```python
from build123d import *

# Parameters (mm, degrees)
SKETCH_1_R           = 30
SKETCH_1_R_2         = 20
EXTRUDE_1_DEPTH      = 30
SKETCH_2_W           = 140
SKETCH_2_H           = 60
EXTRUDE_2_DEPTH      = 10
SKETCH_3_R           = 10
CUT_EXTRUDE_1_DEPTH  = 178.200451467
FILLET_1_RADIUS      = 30
FILLET_1_LENGTH      = 20
EXTRUDE_3_REACH      = 148.287
EXTRUDE_3_END_RADIUS = 30
SKETCH_4_W           = 20
SKETCH_4_H           = 60


with BuildPart() as part:
    # Sketch 1 → Extrude 1 (new, symmetric)
    with BuildSketch(Plane(origin=(0, 0, 0), x_dir=(1, 0, 0), z_dir=(0, 1, 0))):
        with Locations(Location((0, 0, 0), (0, 0, 270))):
            Circle(SKETCH_1_R)
        with Locations(Location((0, 0, 0), (0, 0, 270))):
            Circle(SKETCH_1_R_2, mode=Mode.SUBTRACT)
    extrude(amount=EXTRUDE_1_DEPTH, both=True)



with BuildPart() as body_2:
    # Sketch 2 → Extrude 2 (new, symmetric)
    with BuildSketch(Plane(origin=(0, 0, 0), x_dir=(0, 0, -1), z_dir=(1, 0, 0))):
        with Locations((100, 0)):
            Rectangle(SKETCH_2_W, SKETCH_2_H)
    extrude(amount=EXTRUDE_2_DEPTH, both=True)

    # Sketch 3 → Cut-Extrude 1 (cut, through all)
    with BuildSketch(Plane(origin=(10, 0, 0), x_dir=(0, 0, -1), z_dir=(1, 0, 0))):
        with Locations((140, 0)):
            Circle(SKETCH_3_R)
    extrude(amount=-CUT_EXTRUDE_1_DEPTH, mode=Mode.SUBTRACT)

    # Fillet 1: full round fillet: the end face becomes a half cylinder, R = half its width
    fillet_1_face = Plane((0, 0, -170), x_dir=(1, 0, 0), z_dir=(0, 0, -1))  # on the end face: x along it, z out of the body
    fillet_1_slab = fillet_1_face.offset(-FILLET_1_RADIUS / 2) * Box(FILLET_1_LENGTH, 2 * FILLET_1_RADIUS, FILLET_1_RADIUS, mode=Mode.PRIVATE)  # the body's end, R deep
    fillet_1_round = Plane((0, 0, -140), x_dir=(0, 0, -1), z_dir=(1, 0, 0)) * Cylinder(FILLET_1_RADIUS, FILLET_1_LENGTH, mode=Mode.PRIVATE)  # its axis R under the face
    add(fillet_1_slab - fillet_1_round, mode=Mode.SUBTRACT)


with BuildPart() as part_1:
    add(part.part)

    add(body_2.part)  # Extrude 3 merges body 2
    # Extrude 3: up to this cylinder (the profile starts outside it)
    extrude_3_end = Plane(origin=(0, 0, 0), z_dir=(0, -1, 0)) * Cylinder(EXTRUDE_3_END_RADIUS, 357.574, mode=Mode.PRIVATE)
    # Sketch 4 → Extrude 3 (add, up to the surface)
    with BuildSketch(Plane.XY.offset(-30), mode=Mode.PRIVATE) as extrude_3_sk1:
        Rectangle(SKETCH_4_W, SKETCH_4_H)
    extrude_3_tool1 = extrude(extrude_3_sk1.sketch, amount=EXTRUDE_3_REACH, mode=Mode.PRIVATE) - extrude_3_end
    add(extrude_3_tool1.solids().sort_by_distance((0, 0, -30))[0])
    add(extrude_3_tool1.solids().sort_by_distance((0, 0, -30))[1])


solid = part_1.part
```
Part model, mm, in its own coordinate system. A direction names the side the tool comes from. Give positions to 0.01 mm unless a question says otherwise; leave off trailing zeros. Write each loop counter-clockwise with the first axis right and the second up, starting at its lowest first coordinate (ties: lowest second). Pieces come first, ordered by that corner, then holes. Notation, with made-up numbers: M 13.25,38 L 51.25,38 A21 ccw 51.25,72 Z; hole C -15,-37 d4. An arc over 180 degrees is marked long. Use CSV: the item, a comma, the result in double quotes.
Item 1: Pull direction Y, two halves, no side cores. Call faces 4 (the face through (0.14, -0.66, -169.993)), 5 (the face through (0.14, -3.83, -149.237)), 6 (the face through (0, -30, -56)), 7 (the face through (-19.524, -0.42, -4.336)): +Y half, -Y half, draft (parallel to the pull), parting line (faces both ways), or undercut.
Taken from the geometry:
face 4,"parting line"
face 5,"undercut"
face 6,"-Y half"
face 7,"draft"
Item 2: Drill centre lines: probe 1 along Z at (x, y) = (6.5, 3); probe 2 along Y at (x, z) = (4, -140); probe 3 along X at (y, z) = (13.5, 0). Where is each one in solid material? Low to high.
Taken from the geometry:
probe 1,"z = -169.85 to -149.54, -130.46 to -18.91, 18.91 to 29.29"
probe 2,"y = -30 to -10, 10 to 30"
probe 3,"x = -30 to -20, 20 to 30"
Item 3: Which spindle directions (+Z, -Z, +X, -X, +Y, -Y) get a long thin tool onto all of the face, cutting with end or side? Do faces 1 (the face through (-10, 0, -100)), 2 (the face through (-1.176, 0.42, 29.977)), 3 (the face through (10, 0, -100)). Say none if no direction does.
Taken from the geometry:
face 1,"-Z, -X, +Y, -Y"
face 2,"+Y, -Y"
face 3,"-Z, +X, +Y, -Y"
Item 4: Slice it at C-C on y = 2. Write the cut outline in (x, z).
Taken from the geometry:
outline,"M -10,-169.93 L 10,-169.93 L 10,-149.8 L -10,-149.8 Z; M -10,-130.2 L 10,-130.2 L 10,-28.28 A30 ccw long -10,-28.28 Z; hole C 0,0 d40"
Item 5: Slice it at A-A on x = 0. Write the cut outline in (y, z).
Taken from the geometry:
outline,"M -30,-140 A30 ccw 30,-140 L 30,-20 L -30,-20 Z; M -30,20 L 30,20 L 30,30 L -30,30 Z; hole C 0,-140 d20"
Item 6: Slice it at B-B on z = 0. Write the cut outline in (x, y), plus the area to 3 significant figures.
Taken from the geometry:
outline,"M -30,-30 L -20,-30 L -20,30 L -30,30 Z; M 20,-30 L 30,-30 L 30,30 L 20,30 Z"
area,"1,200 mm²"
Item 7: Slice it at D-D on y = 15. Write the cut outline in (x, z), plus the area to 3 significant figures.
Taken from the geometry:
outline,"M -10,-165.98 L 10,-165.98 L 10,-28.28 A30 ccw long -10,-28.28 Z; hole C 0,0 d40"
area,"4,300 mm²"
Item 8: Pin check, flat tips, straight feed: P1, Ø4, axis at x = -3, y = -16, coming from the -Z side; P2, Ø1, axis at x = 3, y = -2, coming from the +Z side; P3, Ø1, axis at y = -16, z = -24, coming from the -X side. Stop position of each tip, or through.
Taken from the geometry:
P1,"stops at z = -166.53"
P2,"stops at z = 29.9"
P3,"stops at x = -18.65"
